from build123d import *

# Parameters (mm, degrees)
BOSS_EXTRUDE1_DEPTH = 14.47


with BuildPart() as part:
    # Sketch1 → Boss-Extrude1 (new body)
    with BuildSketch(Plane(origin=(0, 0, 0), x_dir=(1, 0, 0), z_dir=(0, 1, 0))):
        Polygon((0, 0), (0, 75.95), (12.7, 75.95), (12.7, 96.4), (137.15, 96.4), (137.15, 94.4), (301.8, 94.4), (301.8, 85.95), (306.92, 85.95), (306.92, 9.15), (301.8, 9.15), (301.8, 0), (155.45, 0), (155.45, 2.35), (150.2, 2.35), (150.2, 0.35), (142.05, 0.35), (142.05, 0), align=None)
    extrude(amount=BOSS_EXTRUDE1_DEPTH)


solid = part.part
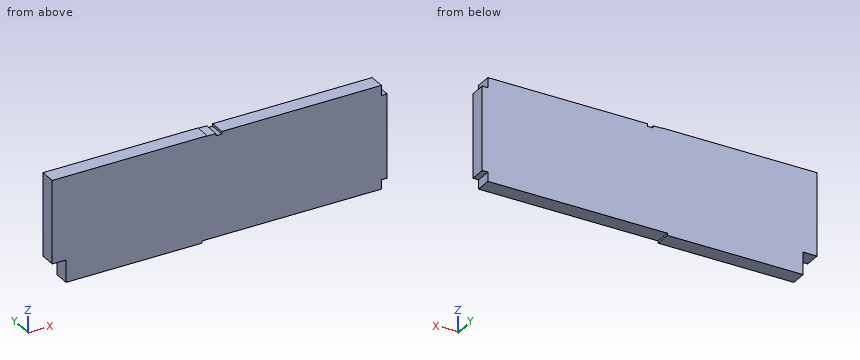
For this review, take the finished solid that the model builds, in its own axes (mm). Give positions to 0.01 mm unless a question says otherwise; leave off trailing zeros. Order: outer loops, then holes, each group sorted by start corner. A loop starts at its lowest first (then second) coordinate and runs counter-clockwise, first axis right, second up. Notation, with made-up numbers: M 61,-25 L 71,-25 A4 cw 71,-20 Z; hole C -26.5,-13.75 d7. An arc over 180 degrees is marked long. Answer in a Markdown table with one row per item. Add a question column.
(1) For pin 1 (1.5 mm diameter, centred on x = 211.5, y = 12.5, fed in from -Z); pin 2 (4 mm diameter, centred on x = 9, y = 9, fed in from -Z); pin 3 (7 mm diameter, centred on y = 4.5, z = -86.5, fed in from -X), all flat-tipped, find the tip position at first contact; note any pin that passes through.
(2) Consider section A-A on y = 6. State the section outline as (x, z) points.
(3) Consider section B-B on z = -80.5. State the section outline as (x, y) points.
(4) Wall thickness on probe 1 along Z at (x, y) = (267.5, 6.5); probe 2 along X at (y, z) = (6.25, -82): over which ranges is each line inside the solid? List them lowest first. Write a range as [from, to].
(5) Consider section C-C on x = 232. State the section outline as (y, z) points.
Evaluation:
| question | item | result |
|---|---|---|
| 1 | pin 1 | stops at z = -94.4 |
| 1 | pin 2 | stops at z = -75.95 |
| 1 | pin 3 | stops at x = 12.7 |
| 2 | outline | M 0,-75.95 L 12.7,-75.95 L 12.7,-96.4 L 137.15,-96.4 L 137.15,-94.4 L 301.8,-94.4 L 301.8,-85.95 L 306.92,-85.95 L 306.92,-9.15 L 301.8,-9.15 L 301.8,0 L 155.45,0 L 155.45,-2.35 L 150.2,-2.35 L 150.2,-0.35 L 142.05,-0.35 L 142.05,0 L 0,0 Z |
| 3 | outline | M 12.7,0 L 306.92,0 L 306.92,14.47 L 12.7,14.47 Z |
| 4 | probe 1 | z = [-94.4, 0] |
| 4 | probe 2 | x = [12.7, 306.92] |
| 5 | outline | M 0,-94.4 L 14.47,-94.4 L 14.47,0 L 0,0 Z |
